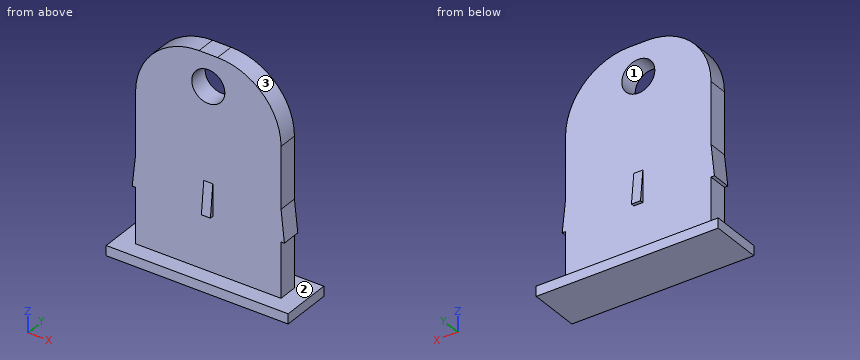
```python
from build123d import *

# Parameters (mm, degrees)
F1_DEPTH       = 2.38125
F2_W           = 34.925
F2_H           = 4.6228
F3_DEPTH       = 50.8
F4_R           = 15.24
F5_R           = 3.96875
F6_DEPTH       = 8.4639625
F8_DEPTH       = 4.6228
F11_DEPTH      = 1.0795
F11_DEPTH_BACK = 1.0922


with BuildPart() as f1:
    # F0 (on Top) → F1 (new body)
    with BuildSketch(Plane.XY):
        Polygon((-21.844, -6.1515625), (21.844, -6.1515625), (21.844, 6.1515625), (-21.844, 6.1515625), align=None)
    extrude(amount=F1_DEPTH)

    # F2 (on face) → F3 (join)
    with BuildSketch(Plane.XY.offset(2.38125)):
        Rectangle(F2_W, F2_H)
    extrude(amount=F3_DEPTH)

    # F4
    f4_edges = [f1.edges().sort_by_distance(p)[0] for p in [
        (-17.4625, 0, 53.18125),
        (17.4625, 0, 53.18125),
    ]]
    fillet(f4_edges, radius=F4_R)

    # F5 (on face) → F6 (cut, through all)
    with BuildSketch(Plane(origin=(0, 2.3114, 0), x_dir=(-1, 0, 0), z_dir=(0, 1, 0))):
        with Locations((0, 45.56125)):
            Circle(F5_R)
    extrude(amount=-F6_DEPTH, mode=Mode.SUBTRACT)

    # F7 (on face) → F8 (join, through all)
    with BuildSketch(Plane.XZ.offset(2.3114)):
        Polygon((18.2753, 15.58925), (17.4625, 23.20925), (17.4625, 15.58925), align=None)
    extrude(amount=-F8_DEPTH)

    # F9: F1 across plane


with BuildPart() as f1_1:
    add(f1.part)
    add(f1.part.mirror(Plane.YZ))

    # F10 (on Right) → F11 (join, two sides)
    with BuildSketch(Plane.YZ) as f11_sk:
        Polygon((-3.1242, 15.58925), (-2.3114, 15.58925), (-2.3114, 23.20925), align=None)
        Polygon((3.1242, 15.58925), (2.3114, 23.20925), (2.3114, 15.58925), align=None)
    extrude(amount=F11_DEPTH)
    extrude(f11_sk.sketch, amount=-F11_DEPTH_BACK)


solid = f1_1.part
```
For this review, take the finished solid that the model builds, in its own axes (mm). Face numbers are marked on the shaded views. Coordinates: 2 decimals unless noted, no trailing zeros. Order: outer loops, then holes, each group sorted by start corner. A loop starts at its lowest first (then second) coordinate and runs counter-clockwise, first axis right, second up. Notation, with made-up numbers: (23.25, 68.25) - (31.25, 68.25) arc R16 cw to (31.25, 84.25) - close; hole circle Ø6 at (47, 82.25). An arc over 180 degrees is marked (long way). Answer as a JSON object with one key per item and string values. Group by question number.
1. We need section C-C on y = 1.25. State the section outline as (x, z) points, then the cut area to 3 significant figures.
2. Clearance check with flat-ended pins moving along their axes: P1, Ø3, axis at x = -9.5, z = 45.5, coming from the -Y side; P2, Ø1.4, axis at y = 0.5, z = 12, coming from the +X side; P3, Ø10, axis at x = 8, z = 26, coming from the +Y side. State where each tip first meets the part, or that it passes through.
3. We need section D-D on x = 19.5. State the section outline as (y, z) points, then the cut area to 3 significant figures.
4. We need section B-B on z = 44.5. State the section outline as (x, y) points, then the cut area to 3 significant figures.
5. The part is to be moulded in two halves that separate along X. For the marked faces 1, 2 and 3, say which applies: pulls with the +X half, pulls with the -X half, needs draft (parallel to the pull), parting line crosses it, or undercut.
6. We need section A-A on x = 0. State the section outline as (y, z) points, then the cut area to 3 significant figures.
7. For probe 1 along Z at (x, y) = (0, 0.1); probe 2 along Z at (x, y) = (7, 3); probe 3 along X at (y, z) = (-2, 35.5), list the stretches that pass through material, from the lowest coordinate up.
Final values:
{
 "1": {"outline": "(-21.84, 0) - (21.84, 0) - (21.84, 2.38) - (17.46, 2.38) - (17.46, 15.59) - (18.28, 15.59) - (17.46, 23.21) - (17.46, 37.94) arc R15.24 ccw to (2.22, 53.18) - (-2.22, 53.18) arc R15.24 ccw to (-17.46, 37.94) - (-17.46, 23.21) - (-18.28, 15.59) - (-17.46, 15.59) - (-17.46, 2.38) - (-21.84, 2.38) - close; hole circle Ø7.94 at (0, 45.56)", "area": "1,740 mm²"},
 "2": {"P1": "y = -2.31", "P2": "x = 17.46", "P3": "y = 2.31"},
 "3": {"outline": "(-6.15, 0) - (6.15, 0) - (6.15, 2.38) - (-6.15, 2.38) - close", "area": "29.3 mm²"},
 "4": {"outline": "(-15.98, -2.31) - (-3.82, -2.31) - (-3.82, 2.31) - (-15.98, 2.31) - close; (3.82, -2.31) - (15.98, -2.31) - (15.98, 2.31) - (3.82, 2.31) - close", "area": "112 mm²"},
 "5": {"face 1": "undercut", "face 2": "needs draft", "face 3": "pulls with the +X half"},
 "6": {"outline": "(-6.15, 0) - (6.15, 0) - (6.15, 2.38) - (2.31, 2.38) - (2.31, 15.59) - (3.12, 15.59) - (2.31, 23.21) - (2.31, 41.59) - (-2.31, 41.59) - (-2.31, 23.21) - (-3.12, 15.59) - (-2.31, 15.59) - (-2.31, 2.38) - (-6.15, 2.38) - close; (-2.31, 49.53) - (2.31, 49.53) - (2.31, 53.18) - (-2.31, 53.18) - close", "area": "234 mm²"},
 "7": {"probe 1": "0 to 41.59, 49.53 to 53.18", "probe 2": "0 to 2.38", "probe 3": "-17.46 to 17.46"}
}
